Source: CAD feature listing. Evaluate the final solid. Frame: model axes, mm. Face numbers are marked on the shaded views. A direction names the side the tool comes from. Give positions to 0.01 mm unless a question says otherwise; leave off trailing zeros. Write each loop counter-clockwise with the first axis right and the second up, starting at its lowest first coordinate (ties: lowest second). Pieces come first, ordered by that corner, then holes.
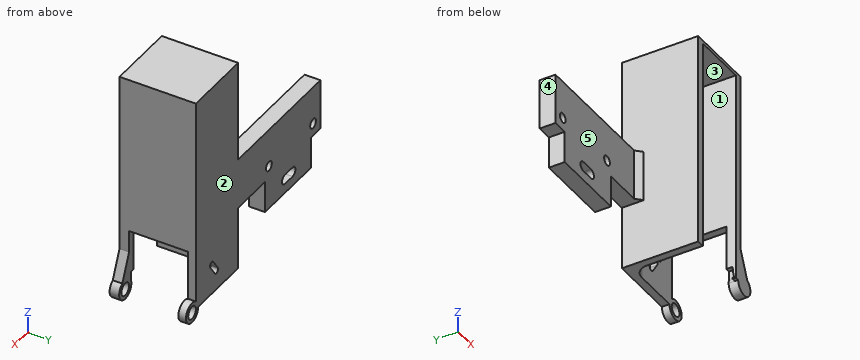
```python
from build123d import *

# Parameters (mm, degrees)
BOSS_EXTRUDE1_DEPTH  = 12.5
BOSS_EXTRUDE2_DEPTH  = 60
SKETCH3_W            = 50
SKETCH3_H            = 55
CUT_EXTRUDE1_DEPTH   = 167.5
FILLET1_SIZE         = 2.5
FILLET1_SIZE_2       = 10
BOSS_EXTRUDE3_REACH  = 196.792
SKETCH6_R            = 7.951814216
CUT_EXTRUDE2_DEPTH   = 55
SKETCH9_W            = 5.049792513
SKETCH9_H            = 55
CUT_EXTRUDE3_DEPTH   = 2.5
SKETCH10_R           = 5
CUT_EXTRUDE4_DEPTH   = 58.5
SKETCH11_W           = 20
SKETCH11_H           = 55
CUT_EXTRUDE6_DEPTH   = 2.5
SKETCH12_W           = 49.615365164
SKETCH12_H           = 4.469133196
CUT_EXTRUDE7_DEPTH   = 167.5
BOSS_EXTRUDE4_START  = 5
SKETCH13_R           = 5
BOSS_EXTRUDE4_DEPTH  = 5
BOSS_EXTRUDE5_DEPTH  = 2.5
SKETCH17_W           = 167.5
SKETCH17_H           = 57.5
BOSS_EXTRUDE6_DEPTH  = 3.5
BOSS_EXTRUDE7_DEPTH  = 3.5
SKETCH20_W           = 139.813438208
SKETCH20_H           = 51.5
BOSS_EXTRUDE8_DEPTH  = 3.5
BOSS_EXTRUDE9_DEPTH  = 3.115365164
BOSS_EXTRUDE10_START = 4
BOSS_EXTRUDE10_DEPTH = 4
SKETCH24_R           = 3.75
CUT_EXTRUDE8_DEPTH   = 210.262529948
CUT_EXTRUDE9_DEPTH   = 210.262529948
SKETCH26_R           = 5
CUT_EXTRUDE10_DEPTH  = 3.5
BOSS_EXTRUDE11_DEPTH = 40
FILLET2_R            = 10
CUT_EXTRUDE11_DEPTH  = 6
SKETCH30_W           = 17.446895317
SKETCH30_H           = 47.5
CUT_EXTRUDE12_DEPTH  = 15
BOSS_EXTRUDE12_START = 1
BOSS_EXTRUDE12_DEPTH = 1


with BuildPart() as part:
    # Sketch1 → Boss-Extrude1 (new body)
    with BuildSketch(Plane(origin=(0, 0, 0), x_dir=(1, 0, 0), z_dir=(0, 1, 0))):
        Polygon((0, 0), (0, 40), (12, 40), (12, 65), (72, 65), (72, 40), (107, 40), (107, 0), align=None)
    extrude(amount=BOSS_EXTRUDE1_DEPTH)

    # Sketch2 → Boss-Extrude2 (add)
    with BuildSketch(Plane(origin=(0, 12.5, 0), x_dir=(1, 0, 0), z_dir=(0, 1, 0))):
        Polygon((107, 0), (107, 40), (107, 90), (162, 90), (162, -80), (107, -80), align=None)
    extrude(amount=-BOSS_EXTRUDE2_DEPTH)

    # Sketch3 → Cut-Extrude1 (cut)
    with BuildSketch(Plane(origin=(0, 0, -90), x_dir=(-1, 0, 0), z_dir=(0, 0, -1))):
        with Locations((-134.5, -17.5)):
            Rectangle(SKETCH3_W, SKETCH3_H)
    extrude(amount=-CUT_EXTRUDE1_DEPTH, mode=Mode.SUBTRACT)

    # Fillet1
    # an asymmetric fillet: 10, 2.5 mm, written as the material it takes off along each edge
    with BuildSketch(Plane(origin=(159.5, -45, -90), x_dir=(0, -1, 0), z_dir=(-1, 0, 0))) as fillet1_piece_1:
        with BuildLine():
            Bezier((FILLET1_SIZE, 0), (0, 0), (0, FILLET1_SIZE_2), weights=[1, 0.707106781, 1])
            Line((0, FILLET1_SIZE_2), (0, 0))
            Line((0, 0), (FILLET1_SIZE, 0))
        make_face()
    extrude(amount=50, mode=Mode.SUBTRACT)

    # Boss-Extrude3: up to this face of the body (flat: up to its plane)
    boss_extrude3_end = Plane(part.part.faces().sort_by_distance((134.5, -47.5, -5))[0])
    # Sketch6 → Boss-Extrude3 (add, up to the picked face)
    with BuildSketch(Plane(origin=(0, 12.5, 0), x_dir=(1, 0, 0), z_dir=(0, 1, 0)), mode=Mode.PRIVATE) as boss_extrude3_sk1:
        with Locations((166.966019237, 90)):
            Circle(SKETCH6_R)
    boss_extrude3_tool1 = split(extrude(boss_extrude3_sk1.sketch, amount=-BOSS_EXTRUDE3_REACH, mode=Mode.PRIVATE), bisect_by=boss_extrude3_end, keep=Keep.BOTH, mode=Mode.PRIVATE)
    add(boss_extrude3_tool1.solids().sort_by(Axis((166.966019, 12.5, -90), (0, -1, 0)))[0])

    # Sketch7 → Cut-Extrude2 (cut)
    with BuildSketch(Plane(origin=(0, 10, 0), x_dir=(1, 0, 0), z_dir=(0, 1, 0))):
        with BuildLine():
            ThreePointArc((162, 83.789524795), (174.132615768, 93.445467092), (159.01420502, 90))
            ThreePointArc((159.01420502, 90), (159.799422705, 86.554532908), (162, 83.789524795))
        make_face()
    extrude(amount=-CUT_EXTRUDE2_DEPTH, mode=Mode.SUBTRACT)

    # Sketch9 → Cut-Extrude3 (cut)
    with BuildSketch(Plane(origin=(162, 0, 0), x_dir=(0, 0, -1), z_dir=(1, 0, 0))):
        with Locations((84.738334464, -17.5)):
            Rectangle(SKETCH9_W, SKETCH9_H)
    extrude(amount=-CUT_EXTRUDE3_DEPTH, mode=Mode.SUBTRACT)

    # Sketch10 → Cut-Extrude4 (cut)
    with BuildSketch(Plane(origin=(0, 12.5, 0), x_dir=(1, 0, 0), z_dir=(0, 1, 0))):
        with Locations(Location((166.966019237, 90, 0), (0, 0, 270))):
            Circle(SKETCH10_R)
    extrude(amount=-CUT_EXTRUDE4_DEPTH, mode=Mode.SUBTRACT)

    # Sketch11 → Cut-Extrude6 (cut)
    with BuildSketch(Plane(origin=(162, 0, 0), x_dir=(0, 0, -1), z_dir=(1, 0, 0))):
        with Locations((72.313438208, -17.5)):
            Rectangle(SKETCH11_W, SKETCH11_H)
    extrude(amount=-CUT_EXTRUDE6_DEPTH, mode=Mode.SUBTRACT)

    # Sketch12 → Cut-Extrude7 (cut)
    with BuildSketch(Plane(origin=(0, 0, -90), x_dir=(-1, 0, 0), z_dir=(0, 0, -1))):
        with Locations((-134.307682582, -47.234566598)):
            Rectangle(SKETCH12_W, SKETCH12_H)
    extrude(amount=-CUT_EXTRUDE7_DEPTH, mode=Mode.SUBTRACT)

    # Sketch13 → Boss-Extrude4 (add)
    with BuildSketch(Plane(origin=(0, -45, 0), x_dir=(1, 0, 0), z_dir=(0, 1, 0)).offset(BOSS_EXTRUDE4_START)):
        with BuildLine():
            ThreePointArc((162, 83.789524795), (174.132615768, 93.445467092), (159.01420502, 90))
            ThreePointArc((159.01420502, 90), (159.799422705, 86.554532908), (162, 83.789524795))
        make_face()
        with Locations(Location((166.966019237, 90, 0), (0, 0, 270))):
            Circle(SKETCH13_R, mode=Mode.SUBTRACT)
    extrude(amount=-BOSS_EXTRUDE4_DEPTH)

    # Sketch15 → Boss-Extrude5 (add)
    with BuildSketch(Plane(origin=(0, -45, 0), x_dir=(1, 0, 0), z_dir=(0, 1, 0))):
        with BuildLine():
            Line((162, 62.313438208), (162, 83.789524795))
            ThreePointArc((162, 83.789524795), (166.263013728, 82.079322467), (170.760595676, 83.011971739))
            Line((170.760595676, 83.011971739), (162, 62.313438208))
        make_face()
    extrude(amount=-BOSS_EXTRUDE5_DEPTH)

    # Sketch17 → Boss-Extrude6 (add)
    with BuildSketch(Plane(origin=(109.5, 0, 0), x_dir=(0, 0, -1), z_dir=(1, 0, 0))):
        with Locations((6.25, -18.75)):
            Rectangle(SKETCH17_W, SKETCH17_H)
    extrude(amount=BOSS_EXTRUDE6_DEPTH)

    # Sketch19 → Boss-Extrude7 (add)
    with BuildSketch(Plane.XZ.offset(-10)):
        with BuildLine():
            Line((159.5, 77.5), (113, 77.5))
            Line((113, 77.5), (113, -90))
            Line((113, -90), (159.01420502, -90))
            ThreePointArc((159.01420502, -90), (174.132615768, -93.445467092), (162, -83.789524795))
            Line((162, -83.789524795), (162, -62.313438208))
            Line((162, -62.313438208), (159.5, -62.313438208))
            Line((159.5, -62.313438208), (159.5, 77.5))
        make_face()
    extrude(amount=BOSS_EXTRUDE7_DEPTH)

    # Sketch20 → Boss-Extrude8 (add)
    with BuildSketch(Plane.ZY.offset(-159.5)):
        with Locations((7.593280896, -19.25)):
            Rectangle(SKETCH20_W, SKETCH20_H)
    extrude(amount=BOSS_EXTRUDE8_DEPTH)

    # Sketch21 → Boss-Extrude9 (add)
    with BuildSketch(Plane.ZY.offset(-159.115365164)):
        with BuildLine():
            Line((-90, -47.5), (77.5, -47.5))
            Line((77.5, -47.5), (77.5, -45))
            Line((77.5, -45), (-62.313438208, -45))
            Line((-62.313438208, -45), (-80, -45))
            add(Edge.make_bspline(
                [(-80, -45), (-85.875836894, -45), (-88.73565038, -46.28323142)],
                knots=[0.331688308, 0.331688308, 0.331688308, 1, 1, 1], degree=2, weights=[1, 0.804256037, 0.870148033]))
            Line((-88.73565038, -46.28323142), (-88.73565038, -45))
            Line((-88.73565038, -45), (-90, -45))
            Line((-90, -45), (-90, -47.5))
        make_face()
    extrude(amount=BOSS_EXTRUDE9_DEPTH)

    # Sketch22 → Boss-Extrude10 (add)
    with BuildSketch(Plane(origin=(0, -45, 0), x_dir=(1, 0, 0), z_dir=(0, 1, 0)).offset(BOSS_EXTRUDE10_START)):
        with BuildLine():
            Line((159.5, 80), (159.115365164, 80))
            Line((159.115365164, 80), (156, 80))
            Line((156, 80), (156, 62.313438208))
            Line((156, 62.313438208), (162, 62.313438208))
            Line((162, 62.313438208), (170.760595676, 83.011971739))
            ThreePointArc((170.760595676, 83.011971739), (164.157429949, 82.560700601), (159.5, 87.263230721))
            Line((159.5, 87.263230721), (159.5, 80))
        make_face()
    extrude(amount=-BOSS_EXTRUDE10_DEPTH)

    # Sketch24 → Cut-Extrude8 (cut, through all)
    with BuildSketch(Plane(origin=(0, 12.5, 0), x_dir=(1, 0, 0), z_dir=(0, 1, 0))):
        with Locations(Location((67, 30, 0), (0, 0, 270))):
            Circle(SKETCH24_R)
        with Locations(Location((9.5, 30, 0), (0, 0, 270))):
            Circle(SKETCH24_R)
    extrude(amount=-CUT_EXTRUDE8_DEPTH, mode=Mode.SUBTRACT)

    # Sketch25 → Cut-Extrude9 (cut, through all)
    with BuildSketch(Plane(origin=(0, 12.5, 0), x_dir=(1, 0, 0), z_dir=(0, 1, 0))):
        with BuildLine():
            Line((36.227939868, 57.5), (46.227939868, 57.5))
            ThreePointArc((46.227939868, 57.5), (49.977939868, 53.75), (46.227939868, 50))
            Line((46.227939868, 50), (36.227939868, 50))
            ThreePointArc((36.227939868, 50), (32.477939868, 53.75), (36.227939868, 57.5))
        make_face()
    extrude(amount=-CUT_EXTRUDE9_DEPTH, mode=Mode.SUBTRACT)

    # Sketch26 → Cut-Extrude10 (cut)
    with BuildSketch(Plane(origin=(0, 10, 0), x_dir=(1, 0, 0), z_dir=(0, 1, 0))):
        with Locations(Location((166.966019237, 90, 0), (0, 0, 270))):
            Circle(SKETCH26_R)
    extrude(amount=-CUT_EXTRUDE10_DEPTH, mode=Mode.SUBTRACT)

    # Sketch27 → Boss-Extrude11 (add)
    with BuildSketch(Plane(origin=(0, 0, -40), x_dir=(-1, 0, 0), z_dir=(0, 0, -1))):
        Polygon((-102.323268395, 0), (-107, -4.676731605), (-107, 0), align=None)
    extrude(amount=-BOSS_EXTRUDE11_DEPTH)

    # Fillet2
    fillet2_edges = [part.edges().sort_by_distance(p)[0] for p in [
        (113, 6.5, -6.25),
        (156, 6.5, 7.593280896),
    ]]
    fillet(fillet2_edges, radius=FILLET2_R)

    # Sketch28 → Cut-Extrude11 (cut)
    with BuildSketch(Plane(origin=(0, 12.5, 0), x_dir=(1, 0, 0), z_dir=(0, 1, 0))):
        with BuildLine():
            Line((137.427240594, 75.66601743), (143.112121915, 67.439102797))
            ThreePointArc((143.112121915, 67.439102797), (142.527454254, 64.239389728), (139.327741185, 64.82405739))
            Line((139.327741185, 64.82405739), (133.642859864, 73.050972022))
            ThreePointArc((133.642859864, 73.050972022), (134.227527525, 76.250685091), (137.427240594, 75.66601743))
        make_face()
    extrude(amount=-CUT_EXTRUDE11_DEPTH, mode=Mode.SUBTRACT)

    # Sketch30 → Cut-Extrude12 (cut)
    with BuildSketch(Plane(origin=(162, 0, 0), x_dir=(0, 0, -1), z_dir=(1, 0, 0))):
        with Locations((53.58999055, -17.25)):
            Rectangle(SKETCH30_W, SKETCH30_H)
    extrude(amount=-CUT_EXTRUDE12_DEPTH, mode=Mode.SUBTRACT)

    # Sketch31 → Boss-Extrude12 (add)
    with BuildSketch(Plane(origin=(0, -41, 0), x_dir=(1, 0, 0), z_dir=(0, 1, 0)).offset(BOSS_EXTRUDE12_START)):
        with BuildLine():
            Line((159.5, 87.263230721), (159.5, 80))
            Line((159.5, 80), (156, 80))
            Line((156, 80), (156, 44.866542891))
            Line((156, 44.866542891), (162, 44.866542891))
            Line((162, 44.866542891), (162, 62.313438208))
            Line((162, 62.313438208), (170.760595676, 83.011971739))
            ThreePointArc((170.760595676, 83.011971739), (164.157429949, 82.560700601), (159.5, 87.263230721))
        make_face()
    extrude(amount=-BOSS_EXTRUDE12_DEPTH)


solid = part.part
```
1. Access query for the marked faces 1 and 2. Directions: +Z, -Z, +X, -X, +Y, -Y. A direction counts if a zero-diameter tool reaches every point of the face in a straight line with its end or side. Return the directions, or none.
2. Section query C-C (y = -36.5). Return loops of the section in (x, z), plus the area to 3 significant figures.
3. Section query B-B (z = -53.75). Return loops of the section in (x, y).
4. Section query A-A (x = 67). Return loops of the section in (y, z).
5. Section query D-D (z = 8). Return loops of the section in (x, y), plus the area to 3 significant figures.
6. Pull-direction query (X, two-part tool) for the marked faces 3, 4 and 5; classes: pulls with the +X half, pulls with the -X half, needs draft (parallel to the pull), parting line crosses it, or undercut.
7. Line query: probe 1 along X at (y, z) = (8, -30); probe 2 along X at (y, z) = (-11.5, 68.5); probe 3 along X at (y, z) = (4.75, -30). Output: solid intervals per line, ascending.
8. Pin query (flat end, axial travel): P1, Ø1.5, axis at y = -30.5, z = -38, coming from the +X side; P2, Ø10, axis at x = 9.5, z = -30, coming from the -Y side; P3, Ø10, axis at y = 1.5, z = -49, coming from the -X side; P4, Ø4.5, axis at x = 67, z = -30, coming from the +Y side. Return the tip coordinate at first contact, or that it passes through.
The answers:
1. face 1: -Z, -Y
1. face 2: +Z, -Z, +X, -X, +Y
2. outline: (107, -90) - (113, -90) - (113, 77.5) - (156, 77.5) - (156, -44.87) - (162, -44.87) - (162, 80) - (107, 80) - close
2. area: 1,880 mm2
3. outline: (12, 0) - (32.48, 0) - (32.48, 12.5) - (12, 12.5) - close; (49.98, 0) - (72, 0) - (72, 12.5) - (49.98, 12.5) - close; (107, -47.5) - (113, -47.5) - (113, -3.5) arc R10 cw to (123, 6.5) - (146, 6.5) arc R10 cw to (147, 6.45) - (147, 6.5) - (162, 6.5) - (162, 12.5) - (107, 12.5) - close; (156, -47.5) - (162, -47.5) - (162, -40) - (156, -40) - close
4. outline: (0, -65) - (12.5, -65) - (12.5, -33.75) - (0, -33.75) - close; (0, -26.25) - (12.5, -26.25) - (12.5, 0) - (0, 0) - close
5. outline: (107, -47.5) - (113, -47.5) - (113, -3.5) arc R10 cw to (123, 6.5) - (146, 6.5) arc R10 cw to (156, -3.5) - (156, -47.5) - (162, -47.5) - (162, 12.5) - (107, 12.5) - close
5. area: 1,020 mm2
6. face 3: undercut
6. face 4: pulls with the -X half
6. face 5: needs draft
7. probe 1: x = 0 to 5.75, 13.25 to 63.25, 70.75 to 162
7. probe 2: x = 107 to 113, 156 to 162
7. probe 3: x = 0 to 5.75, 13.25 to 63.25, 70.75 to 117.35, 151.65 to 162
8. P1: stops at x = 162
8. P2: stops at y = 0
8. P3: stops at x = 12
8. P4: passes through
